Could you check a few things on this model? Use its own coordinates, in mm. A direction names the side the tool comes from. Give positions to 0.01 mm unless a question says otherwise; leave off trailing zeros. Use a Markdown table: item, result. Add a question column.
Item 1: If I drill on L1, parallel to Z at x = -11, y = 22 (1 decimal); L2, parallel to Y at x = -9, z = -12.5; L3, parallel to Z at x = -7, y = 21 (1 decimal), over which ranges is the centre line in solid material (lowest first)? Write a range as from..to.
Item 2: If we mould it in two halves opening along Z, with no side actions, what happens to faces 1 (the face through (-4, 19.05, -4)), 2 (the face through (0, 12, 15.875)), 3 (the face through (0, 12, -15.875))? For each: released by +Z, released by -Z, zero draft, split by the parting line, or undercut.
Item 3: I'm going to push a flat-ended pin straight in: pin 1 Ø1.5 at (x, z) = (7.5, -0.5) entering from +Y. Where does the tip first touch, or does it pass through?
Item 4: For faces 4 (the face through (-13, 21, -9.208)), 5 (the face through (-9.208, 21, -12)), 6 (the face through (-13, 23.812, -13)), which set-ups out of +Z, -Z, +X, -X, +Y, -Y let a thin tool reach every point of the face, with its end or its side?
from build123d import *

# Parameters (mm, degrees)
SKETCH1_W           = 31.75
SKETCH1_H           = 31.75
BOSS_EXTRUDE1_DEPTH = 19.05
SKETCH2_W           = 6.6675
SKETCH2_H           = 6.6675
BOSS_EXTRUDE2_DEPTH = 4.7625


with BuildPart() as part:
    # Sketch1 → Boss-Extrude1 (new body)
    with BuildSketch(Plane(origin=(0, 0, 0), x_dir=(1, 0, 0), z_dir=(0, 1, 0))):
        Rectangle(SKETCH1_W, SKETCH1_H)
    extrude(amount=BOSS_EXTRUDE1_DEPTH)

    # Sketch2 → Boss-Extrude2 (add)
    with BuildSketch(Plane(origin=(0, 19.05, 0), x_dir=(1, 0, 0), z_dir=(0, 1, 0))):
        with Locations((-12.54125, 12.54125)):
            Rectangle(SKETCH2_W, SKETCH2_H)
        Polygon((-15.875, -9.2075), (9.2075, -9.2075), (9.2075, 15.875), (15.875, 15.875), (15.875, -15.875), (-15.875, -15.875), align=None)
    extrude(amount=BOSS_EXTRUDE2_DEPTH)


solid = part.part
Findings below:
| question | item | result |
|---|---|---|
| 1 | L1 | z = -15.9..-9.2, 9.2..15.9 |
| 1 | L2 | y = 0..19.05 |
| 1 | L3 | z = 9.2..15.9 |
| 2 | face 1 | undercut |
| 2 | face 2 | released by +Z |
| 2 | face 3 | released by -Z |
| 3 | pin 1 | stops at y = 19.05 |
| 4 | face 4 | -X, +Y |
| 4 | face 5 | -Z, +Y |
| 4 | face 6 | +Z, -Z, +X, -X, +Y |
